Part model, mm, in its own coordinate system. Round coordinates to 2 decimals unless told otherwise and drop trailing zeros. Loops run counter-clockwise (first coordinate to the right, second up) from the corner with the lowest first, then second, coordinate; pieces in that order, holes last. Notation, with made-up numbers: (64, 27.5) -> (86, 27.5) arc R21 cw to (86, 59.5) -> close; hole circle Ø3 at (62, 33). An arc over 180 degrees is marked (long way). Answer as a JSON object with one key per item and string values. Group by question number.
from build123d import *

# Parameters (mm, degrees)
SKETCH1_R             = 15
SKETCH1_R_2           = 1.8288
SKETCH1_R_3           = 11.1125
BOSS_EXTRUDE1_DEPTH   = 3.175
CUT_EXTRUDE1_REACH    = 168.331
SKETCH2_W             = 4.112404804
SKETCH2_H             = 127.6975
FILLET3_R             = 2.5
FILLET4_R             = 10
F_6_CLEARANCE_HOLE1_D = 3.7973


with BuildPart() as part:
    # Sketch1 → Boss-Extrude1 (new body)
    with BuildSketch(Plane(origin=(0, 0, 0), x_dir=(0, 0, -1), z_dir=(1, 0, 0))):
        with BuildLine():
            Line((20.757404804, -103.81), (20.757404804, -5))
            Line((20.757404804, -5), (10.169330134, 22.502104942))
            ThreePointArc((10.169330134, 22.502104942), (16.03292259, 36.599390347), (7.5, 49.260527909))
            Line((7.5, 49.260527909), (7.5, 126.459503782))
            ThreePointArc((7.5, 126.459503782), (0, 165), (-7.5, 126.459503782))
            Line((-7.5, 126.459503782), (-7.5, 49.260527909))
            ThreePointArc((-7.5, 49.260527909), (-16.03292259, 36.599390347), (-10.169330134, 22.502104942))
            Line((-10.169330134, 22.502104942), (-20.757404804, -5))
            Line((-20.757404804, -5), (-20.757404804, -103.81))
            Line((-20.757404804, -103.81), (20.757404804, -103.81))
        make_face()
        with Locations((0, 145)):
            Circle(SKETCH1_R, mode=Mode.SUBTRACT)
        with Locations((-13.4747, -100)):
            Circle(SKETCH1_R_2, mode=Mode.SUBTRACT)
        with Locations((13.4747, -100)):
            Circle(SKETCH1_R_2, mode=Mode.SUBTRACT)
        with Locations((-13.4747, 0)):
            Circle(SKETCH1_R_2, mode=Mode.SUBTRACT)
        with Locations((13.4747, 0)):
            Circle(SKETCH1_R_2, mode=Mode.SUBTRACT)
        with Locations((0, 35)):
            Circle(SKETCH1_R_3, mode=Mode.SUBTRACT)
    extrude(amount=BOSS_EXTRUDE1_DEPTH)

    # Sketch2 → Cut-Extrude1 (cut, up to next)
    with BuildSketch(Plane(origin=(3.175, 0, 0), x_dir=(0, 0, -1), z_dir=(1, 0, 0)), mode=Mode.PRIVATE) as cut_extrude1_sk1:
        Polygon((11.645, -5), (-11.645, -5), (11.645, -27.976379872), align=None)
    cut_extrude1_tool1 = extrude(cut_extrude1_sk1.sketch, amount=-CUT_EXTRUDE1_REACH, mode=Mode.PRIVATE) & part.part
    # Sketch2 → Cut-Extrude1 (cut, up to next)
    with BuildSketch(Plane(origin=(3.175, 0, 0), x_dir=(0, 0, -1), z_dir=(1, 0, 0)), mode=Mode.PRIVATE) as cut_extrude1_sk2:
        Polygon((-11.645, -12.023620128), (11.645, -35), (-11.645, -57.976379872), (-11.645, -35), align=None)
    cut_extrude1_tool2 = extrude(cut_extrude1_sk2.sketch, amount=-CUT_EXTRUDE1_REACH, mode=Mode.PRIVATE) & part.part
    # Sketch2 → Cut-Extrude1 (cut, up to next)
    with BuildSketch(Plane(origin=(3.175, 0, 0), x_dir=(0, 0, -1), z_dir=(1, 0, 0)), mode=Mode.PRIVATE) as cut_extrude1_sk3:
        Polygon((-11.645, -72.023620128), (-11.645, -95), (11.645, -95), align=None)
    cut_extrude1_tool3 = extrude(cut_extrude1_sk3.sketch, amount=-CUT_EXTRUDE1_REACH, mode=Mode.PRIVATE) & part.part
    # Sketch2 → Cut-Extrude1 (cut, up to next)
    with BuildSketch(Plane(origin=(3.175, 0, 0), x_dir=(0, 0, -1), z_dir=(1, 0, 0)), mode=Mode.PRIVATE) as cut_extrude1_sk4:
        Polygon((11.645, -42.023620128), (11.645, -65), (11.645, -87.976379872), (-11.645, -65), align=None)
    cut_extrude1_tool4 = extrude(cut_extrude1_sk4.sketch, amount=-CUT_EXTRUDE1_REACH, mode=Mode.PRIVATE) & part.part
    # Sketch2 → Cut-Extrude1 (cut, up to next)
    with BuildSketch(Plane(origin=(3.175, 0, 0), x_dir=(0, 0, -1), z_dir=(1, 0, 0)), mode=Mode.PRIVATE) as cut_extrude1_sk5:
        with Locations((-18.701202402, -39.96125)):
            Rectangle(SKETCH2_W, SKETCH2_H)
    cut_extrude1_tool5 = extrude(cut_extrude1_sk5.sketch, amount=-CUT_EXTRUDE1_REACH, mode=Mode.PRIVATE) & part.part
    # Sketch2 → Cut-Extrude1 (cut, up to next)
    with BuildSketch(Plane(origin=(3.175, 0, 0), x_dir=(0, 0, -1), z_dir=(1, 0, 0)), mode=Mode.PRIVATE) as cut_extrude1_sk6:
        with Locations((18.701202402, -39.96125)):
            Rectangle(SKETCH2_W, SKETCH2_H)
    cut_extrude1_tool6 = extrude(cut_extrude1_sk6.sketch, amount=-CUT_EXTRUDE1_REACH, mode=Mode.PRIVATE) & part.part
    add(cut_extrude1_tool1.solids().sort_by_distance((3.175, -12.658793, -3.881667))[0], mode=Mode.SUBTRACT)
    add(cut_extrude1_tool2.solids().sort_by_distance((3.175, -35, 3.881667))[0], mode=Mode.SUBTRACT)
    add(cut_extrude1_tool3.solids().sort_by_distance((3.175, -87.341207, 3.881667))[0], mode=Mode.SUBTRACT)
    add(cut_extrude1_tool4.solids().sort_by_distance((3.175, -65, -3.881667))[0], mode=Mode.SUBTRACT)
    add(cut_extrude1_tool5.solids().sort_by_distance((3.175, -39.96125, 18.701202))[0], mode=Mode.SUBTRACT)
    add(cut_extrude1_tool6.solids().sort_by_distance((3.175, -39.96125, -18.701202))[0], mode=Mode.SUBTRACT)

    # Fillet3
    fillet3_edges = [part.edges().sort_by_distance(p)[0] for p in [
        (1.5875, -103.81, -16.645),
        (1.5875, -72.023620128, 11.645),
        (1.5875, -95, -11.645),
        (1.5875, -95, 11.645),
        (1.5875, -87.976379872, -11.645),
        (1.5875, -65, 11.645),
        (1.5875, -42.023620128, -11.645),
        (1.5875, -27.976379872, -11.645),
        (1.5875, -5, 11.645),
        (1.5875, -5, -11.645),
        (1.5875, -103.81, 16.645),
        (1.5875, -12.023620128, 11.645),
        (1.5875, -35, -11.645),
        (1.5875, -57.976379872, 11.645),
    ]]
    fillet(fillet3_edges, radius=FILLET3_R)

    # Fillet4
    fillet4_edges = [part.edges().sort_by_distance(p)[0] for p in [
        (1.5875, 5.681808734, -16.645),
        (1.5875, 22.502104942, 10.169330134),
        (1.5875, 49.260527909, 7.5),
        (1.5875, 126.459503782, 7.5),
        (1.5875, 126.459503782, -7.5),
        (1.5875, 49.260527909, -7.5),
        (1.5875, 22.502104942, -10.169330134),
        (1.5875, 5.681808734, 16.645),
    ]]
    fillet(fillet4_edges, radius=FILLET4_R)

    # #6 Clearance Hole1 (through all)
    with Locations(Plane(origin=(3.175, 0, 0), x_dir=(0, 0, -1), z_dir=(1, 0, 0))):
        with Locations((0, 90)):
            Hole(F_6_CLEARANCE_HOLE1_D / 2)


solid = part.part
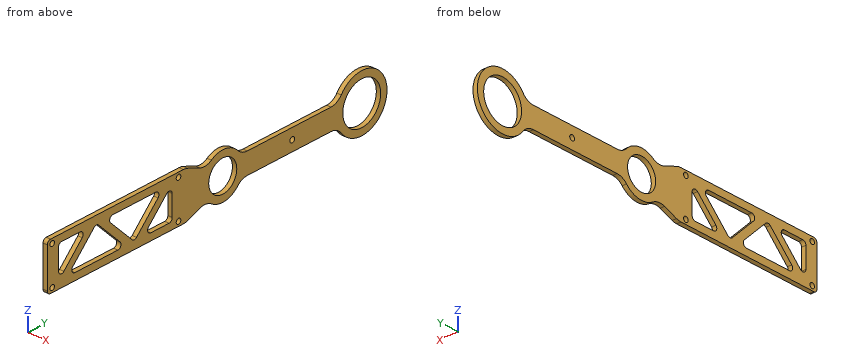
Item 1: Band-saw the part on B-B, the plane x = 2.1. Count the separate pieces of the cut face and the enclosed holes in it, plus the area to 3 significant figures.
Item 2: Drop flat-ended pins along their axis: pin 1 Ø1 at (x, y) = (1, -62.5) entering from +Z (3 decimals); pin 2 Ø1 at (x, y) = (1.5, 76.5) entering from -Z; pin 3 Ø1 at (x, y) = (1, 92) entering from +Z. Give the stop position or say it passes through.
Item 3: Band-saw the part on C-C, the plane y = 108.5. List the corners of the cut face in (x, z) (3 decimals).
Item 4: Band-saw the part on A-A, the plane y = 35. List the corners of the cut face in (x, z) (1 decimal).
Item 5: Drill centre lines: line 1 (Z direction, x = 1.1, y = 90); line 2 (Z direction, x = 1.6, y = 138) (1 decimal); line 3 (Z direction, x = 1.7, y = 10). Where is each one in solid material? Low to high.
Entries:
{
 "1": {"separate pieces": "1", "enclosed holes": "11", "area": "4,580 mm²"},
 "2": {"pin 1": "z = 16.645", "pin 2": "z = -7.5", "pin 3": "z = 7.5"},
 "3": {"outline": "(0, -7.5) -> (3.175, -7.5) -> (3.175, 7.5) -> (0, 7.5) -> close"},
 "4": {"outline": "(0, -16.1) -> (3.2, -16.1) -> (3.2, -11.1) -> (0, -11.1) -> close; (0, 11.1) -> (3.2, 11.1) -> (3.2, 16.1) -> (0, 16.1) -> close"},
 "5": {"line 1": "-7.5 to -1.9, 1.9 to 7.5", "line 2": "-18.7 to -13.3, 13.3 to 18.7", "line 3": "-14.98 to 14.98"}
}
